Model file for the job. Use its own axes, mm. A direction names the side the tool comes from. Round coordinates to 2 decimals unless told otherwise and drop trailing zeros. Order: outer loops, then holes, each group sorted by start corner. A loop starts at its lowest first (then second) coordinate and runs counter-clockwise, first axis right, second up. Notation, with made-up numbers: (74.25, -2) - (121.25, -2) arc R22 ccw to (121.25, 19) - close; hole circle Ø9 at (86.5, 35). An arc over 180 degrees is marked (long way). Write item = value, one per line. Start each with the question number.
from build123d import *

# Parameters (mm, degrees)
SALIENTE_EXTRUIR1_DEPTH = 15
SALIENTE_EXTRUIR2_START = -9
CROQUIS2_W              = 30
CROQUIS2_H              = 11
SALIENTE_EXTRUIR2_DEPTH = 3
SALIENTE_EXTRUIR3_START = 3.5
CROQUIS3_W              = 30
CROQUIS3_H              = 11
SALIENTE_EXTRUIR3_DEPTH = 3
CROQUIS4_R              = 4.5
CORTAR_EXTRUIR1_DEPTH   = 22.914607001
REDONDEO6_R             = 5.5
REDONDEO7_R             = 5.5


with BuildPart() as part:
    # Croquis1 → Saliente-Extruir1 (new body)
    with BuildSketch(Plane(origin=(0, 0, 0), x_dir=(1, 0, 0), z_dir=(0, 1, 0))):
        with BuildLine():
            Line((-5.5, 0), (-5.5, 5.5))
            Line((-5.5, 5.5), (5.5, 5.5))
            Line((5.5, 5.5), (5.5, 0))
            ThreePointArc((5.5, 0), (0, -5.5), (-5.5, 0))
        make_face()
    extrude(amount=SALIENTE_EXTRUIR1_DEPTH)

    # Croquis2 → Saliente-Extruir2 (add)
    with BuildSketch(Plane(origin=(0, 15, 0), x_dir=(1, 0, 0), z_dir=(0, 1, 0)).offset(SALIENTE_EXTRUIR2_START)):
        Rectangle(CROQUIS2_W, CROQUIS2_H)
    extrude(amount=-SALIENTE_EXTRUIR2_DEPTH)

    # Croquis3 → Saliente-Extruir3 (add)
    with BuildSketch(Plane(origin=(0, 6, 0), x_dir=(1, 0, 0), z_dir=(0, 1, 0)).offset(SALIENTE_EXTRUIR3_START)):
        Rectangle(CROQUIS3_W, CROQUIS3_H)
    extrude(amount=SALIENTE_EXTRUIR3_DEPTH)

    # Croquis4 → Cortar-Extruir1 (cut, through all)
    with BuildSketch(Plane(origin=(0, 15, 0), x_dir=(1, 0, 0), z_dir=(0, 1, 0))):
        with Locations(Location((0, 0, 0), (0, 0, 270))):
            Circle(CROQUIS4_R)
    extrude(amount=-CORTAR_EXTRUIR1_DEPTH, mode=Mode.SUBTRACT)

    # Redondeo6
    redondeo6_edges = [part.edges().sort_by_distance(p)[0] for p in [
        (-5.5, 7.75, -5.5),
    ]]
    fillet(redondeo6_edges, radius=REDONDEO6_R - 0.0001)  # a hair under: the kernel refuses the full size

    # Redondeo7
    redondeo7_edges = [part.edges().sort_by_distance(p)[0] for p in [
        (5.5, 7.75, -5.5),
    ]]
    fillet(redondeo7_edges, radius=REDONDEO7_R - 0.0001)  # a hair under: the kernel refuses the full size


solid = part.part
Item 1: Saw through at A-A, the plane x = -9.75. Give the cut face in (y, z), then the cut area to 3 significant figures.
Item 2: Saw through at C-C, the plane z = 0.5. Give the cut face in (x, y), then the cut area to 3 significant figures.
Item 3: Saw through at D-D, the plane y = 3.5. Give the cut face in (x, z), then the cut area to 3 significant figures.
Item 4: Mould opens along Y. For faces 1 (the face through (15, 11, 0)), 2 (the face through (9, 9.5, 0)), 3 (the face through (3, 0, -4)) say: +Y half, -Y half, draft (parallel to the pull), parting line (faces both ways), or undercut.
Item 5: Which spindle directions (+Z, -Z, +X, -X, +Y, -Y) get a long thin tool onto all of the face, cutting with end or side? Do faces 4 (the face through (-5.5, 1, -3)), 5 (the face through (5.5, 14, -3)), 6 (the face through (3.85, 7.77, -3.93)), 7 (the face through (0.1, 1.5, 5.5)). Say none if no direction does.
Item 6: Drop flat-ended pins along their axis: pin 1 (1.2 mm diameter, centred on y = 13.5, z = -4, fed in from -X); pin 2 (1.5 mm diameter, centred on x = 10.5, z = -1, fed in from +Y); pin 3 (0.8 mm diameter, centred on y = 13.5, z = -3, fed in from +X). Give the stop position or say it passes through.
Item 7: Probe L1, parallel to X at y = 8.5, z = 0; L2, parallel to Y at x = -11.75, z = 4; L3, parallel to Y at x = -5.25, z = -3. List the from-to ranges inside material, lowest first.
Check sheet entries:
q1.outline = (3, -5.5) - (6, -5.5) - (6, 5.5) - (3, 5.5) - close; (9.5, -5.5) - (12.5, -5.5) - (12.5, 5.5) - (9.5, 5.5) - close
q1.area = 66.0 mm2
q2.outline = (-15, 3) - (-5.48, 3) - (-5.48, 0) - (-4.47, 0) - (-4.47, 15) - (-5.48, 15) - (-5.48, 12.5) - (-15, 12.5) - (-15, 9.5) - (-5.48, 9.5) - (-5.48, 6) - (-15, 6) - close; (4.47, 0) - (5.48, 0) - (5.48, 3) - (15, 3) - (15, 6) - (5.48, 6) - (5.48, 9.5) - (15, 9.5) - (15, 12.5) - (5.48, 12.5) - (5.48, 15) - (4.47, 15) - close
q2.area = 144 mm2
q3.outline = (-15, -5.5) - (15, -5.5) - (15, 5.5) - (-15, 5.5) - close; hole circle Ø9 at (0, 0)
q3.area = 266 mm2
q4.face_1 = draft
q4.face_2 = undercut
q4.face_3 = -Y half
q5.face_4 = +Z, -Z, -X, -Y
q5.face_5 = +Z, -Z, +X, +Y
q5.face_6 = -Z, +X
q5.face_7 = +Z, -Y
q6.pin_1 = -5.5
q6.pin_2 = 12.5
q6.pin_3 = 5.5
q7.L1 = -5.5 to -4.5, 4.5 to 5.5
q7.L2 = 3 to 6, 9.5 to 12.5
q7.L3 = 0 to 6, 9.5 to 15
